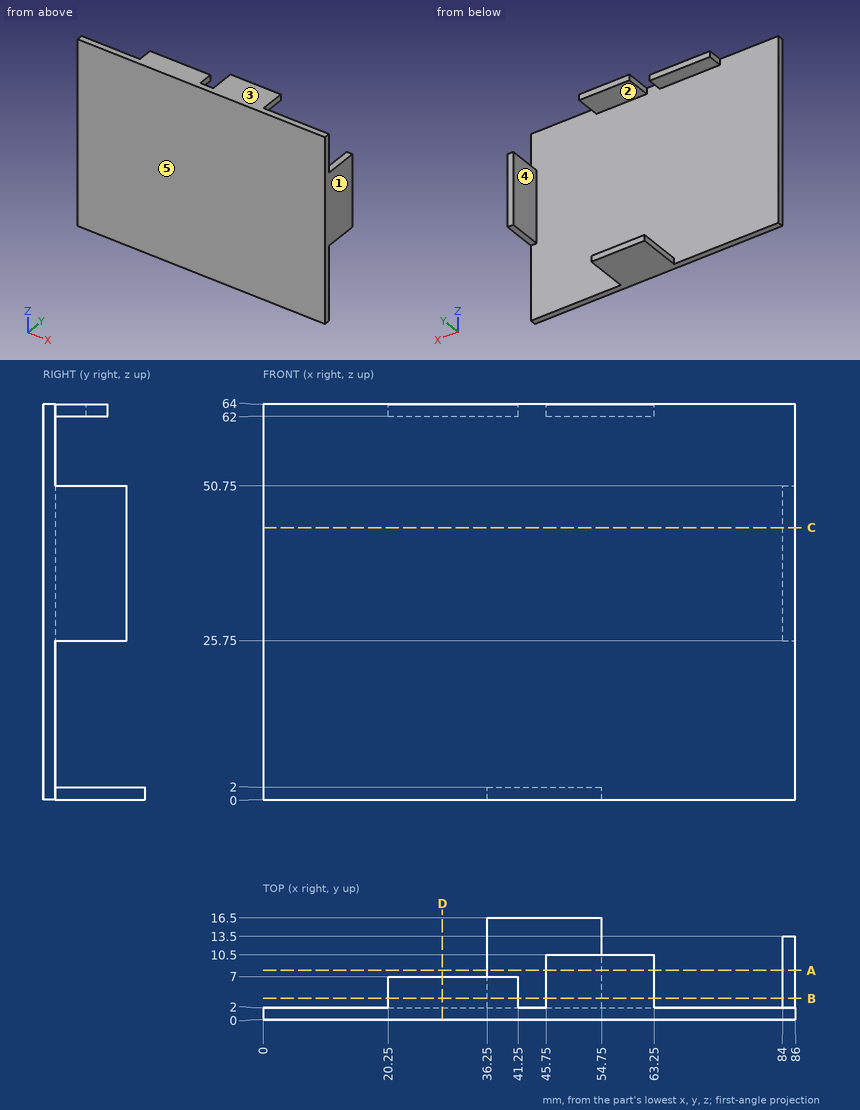
Verification items for this drawing (mm, ordinates from the low corner). A direction names the side the tool comes from. Coordinates: 2 decimals unless noted, no trailing zeros. Order: outer loops, then holes, each group sorted by start corner. A loop starts at its lowest first (then second) coordinate and runs counter-clockwise, first axis right, second up. Notation, with made-up numbers: M 44,-9 L 93,-9 A20 cw 93,21 Z; hole C -2.5,-39 d6. An arc over 180 degrees is marked long. Answer as a JSON object with one key per item and string values.
Q1. Cross-section at B-B on y = 3.5. Record the cut outline in (x, z), and give its area (3 significant figures).
Results are:
{"outline": "M 20.25,62 L 41.25,62 L 41.25,64 L 20.25,64 Z; M 36.25,0 L 54.75,0 L 54.75,2 L 36.25,2 Z; M 45.75,62 L 63.25,62 L 63.25,64 L 45.75,64 Z; M 84,25.75 L 86,25.75 L 86,50.75 L 84,50.75 Z", "area": "164 mm²"}
Q2. Cross-section at A-A on y = 8. Record the cut outline in (x, z).
Results are:
{"outline": "M 36.25,0 L 54.75,0 L 54.75,2 L 36.25,2 Z; M 45.75,62 L 63.25,62 L 63.25,64 L 45.75,64 Z; M 84,25.75 L 86,25.75 L 86,50.75 L 84,50.75 Z"}
Q3. Cross-section at D-D on x = 29. Record the cut outline in (y, z), and give its area (3 significant figures).
Results are:
{"outline": "M 0,0 L 2,0 L 2,62 L 7,62 L 7,64 L 0,64 Z", "area": "138 mm²"}
Q4. Depth check by flat-ended pin: pin 1 Ø5 at (x, z) = (62.5, 33) entering from +Y; pin 2 Ø8 at (x, y) = (70, 7.5) entering from -Z; pin 3 Ø1 at (x, y) = (85.5, 10) entering from +Z; pin 4 Ø3.5 at (y, z) = (10, 42.5) entering from -X. Enter the tip coordinate at first touch or a pass-through.
Results are:
{"pin 1": "stops at y = 2", "pin 2": "passes through", "pin 3": "stops at z = 50.75", "pin 4": "stops at x = 84"}
Q5. Tool access check on the marked faces 4 and 5. Record the directions out of +Z, -Z, +X, -X, +Y, -Y that give a thin tool (end or side, any length) a straight path to the whole face; none if there is none.
Results are:
{"face 4": "+Z, -Z, -X, +Y", "face 5": "+Z, -Z, +X, -X, -Y"}
Q6. Scan lines: line 1 (X direction, y = 3, z = 33); line 2 (Y direction, x = 68.5, z = 54); line 3 (Z direction, x = 63, y = 5.75). Record each from-to range of solid material in increasing order.
Results are:
{"line 1": "x = 84 to 86", "line 2": "y = 0 to 2", "line 3": "z = 62 to 64"}
Q7. Release check for a two-part mould opening along Z. For the marked faces 1, 2 and 3 record: released by +Z, released by -Z, zero draft, split by the parting line, or undercut.
Results are:
{"face 1": "zero draft", "face 2": "undercut", "face 3": "released by +Z"}
Q8. Cross-section at C-C on z = 44. Record the cut outline in (x, y), and give its area (3 significant figures).
Results are:
{"outline": "M 0,0 L 86,0 L 86,13.5 L 84,13.5 L 84,2 L 0,2 Z", "area": "195 mm²"}
